Work out the finished part from the listing and answer in its coordinate system (mm). Face numbers are marked on the shaded views. A direction names the side the tool comes from. Give positions to 0.01 mm unless a question says otherwise; leave off trailing zeros. Loops run counter-clockwise (first coordinate to the right, second up) from the corner with the lowest first, then second, coordinate; pieces in that order, holes last. Notation, with made-up numbers: (63, 65) - (112, 65) arc R15 ccw to (112, 71) - close; hole circle Ø3 at (54.5, -2.75). An arc over 180 degrees is marked (long way). One line per item, written item: value.
from build123d import *

# Parameters (mm, degrees)
PROFILE_EXTRUDE_DEPTH                = 80
SPROCKET_SKETCH_R                    = 0.35
SPROCKET_EXTRUDE_DEPTH               = 1
SPROCKET_PATTERN_COUNT               = 7
SPROCKET_PATTERN_PITCH               = 12
MAGNET_START                         = -6.5
MAGNET_CUT_DEPTH                     = 5
MAGNET_CHAMFER_SIZE                  = 0.75
MAGNET_CHAMFER_OF_MAGNET_MIRROR_SIZE = 0.75


with BuildPart() as part:
    # Profile Sketch → Profile Extrude (new body)
    with BuildSketch(Plane(origin=(0.045617437, 0, -0.024209872), x_dir=(-1, 0, 0), z_dir=(0, 1, 0))):
        Polygon((3.545617437, -11.975790128), (3.545617437, 0.024209872), (-0.104382563, 0.024209872), (-0.104382563, 1.024209872), (-0.954382563, 1.024209872), (-0.954382563, -18.475790128), (13.045617437, -18.475790128), (13.045617437, 1.024209872), (12.195617437, 1.024209872), (12.195617437, 0.024209872), (10.795617437, 0.024209872), (10.795617437, -11.975790128), align=None)
    extrude(amount=PROFILE_EXTRUDE_DEPTH)

    # Sprocket Sketch → Sprocket Extrude (add)
    with BuildSketch(Plane.XY):
        with Locations(Location((-1.75, 2, 0), (0, 0, 180))):
            Circle(SPROCKET_SKETCH_R)
    sprocket_extrude = extrude(amount=SPROCKET_EXTRUDE_DEPTH)

    # Sprocket Pattern: Sprocket Extrude ×7
    with Locations(*[(0, i * SPROCKET_PATTERN_PITCH, 0) for i in range(1, SPROCKET_PATTERN_COUNT)]):
        add(sprocket_extrude)

    # Magnet Hole Sketch → Magnet Cut (cut)
    with BuildSketch(Plane.XY.offset(-12).offset(MAGNET_START)):
        with BuildLine():
            ThreePointArc((-5.276039281, 12.971757773), (-6.369559557, 12.644203044), (-7.125, 13.5))
            ThreePointArc((-7.125, 13.5), (-8.753920776, 14.461963369), (-9.379949311, 12.676789795))
            ThreePointArc((-9.379949311, 12.676789795), (-9.4063426, 11.535570233), (-10.453697807, 11.08155948))
            ThreePointArc((-10.453697807, 11.08155948), (-11.87194354, 9.829626791), (-10.367596036, 8.682589301))
            ThreePointArc((-10.367596036, 8.682589301), (-9.29038771, 8.304831552), (-9.182248383, 7.16844052))
            ThreePointArc((-9.182248383, 7.16844052), (-8.429851675, 5.432740197), (-6.874085251, 6.509005616))
            ThreePointArc((-6.874085251, 6.509005616), (-6.181940604, 7.41675805), (-5.067751617, 7.16844052))
            ThreePointArc((-5.067751617, 7.16844052), (-3.184499145, 7.347651415), (-3.727330121, 9.159857515))
            ThreePointArc((-3.727330121, 9.159857515), (-4.37676953, 10.098637121), (-3.796302193, 11.08155948))
            ThreePointArc((-3.796302193, 11.08155948), (-3.384784865, 12.928018228), (-5.276039281, 12.971757773))
        make_face()
    magnet_cut = extrude(amount=MAGNET_CUT_DEPTH, mode=Mode.SUBTRACT)

    # Magnet Chamfer
    magnet_chamfer_edges = [part.edges().sort_by_distance(p)[0] for p in [
        (-3.384784865, 12.928018228, -18.5),
        (-8.753920776, 14.461963369, -18.5),
        (-11.87194354, 9.829626791, -18.5),
        (-8.429851675, 5.432740197, -18.5),
        (-3.184499145, 7.347651415, -18.5),
        (-4.37676953, 10.098637121, -18.5),
        (-6.181940604, 7.41675805, -18.5),
        (-9.29038771, 8.304831552, -18.5),
        (-9.4063426, 11.535570233, -18.5),
        (-6.369559557, 12.644203044, -18.5),
    ]]
    chamfer(magnet_chamfer_edges, length=MAGNET_CHAMFER_SIZE)

    # Magnet Mirror: Magnet Cut across plane
    add(magnet_cut.mirror(Plane(origin=(0, 40, 0), x_dir=(0, 0, 1), z_dir=(0, -1, 0))), mode=Mode.SUBTRACT)

    # Magnet Chamfer of Magnet Mirror
    magnet_chamfer_of_magnet_mirror_edges = [part.edges().sort_by_distance(p)[0] for p in [
        (-3.384784865, 67.071981772, -18.5),
        (-8.753920776, 65.538036631, -18.5),
        (-11.87194354, 70.170373209, -18.5),
        (-8.429851675, 74.567259803, -18.5),
        (-3.184499145, 72.652348585, -18.5),
        (-4.37676953, 69.901362879, -18.5),
        (-6.181940604, 72.58324195, -18.5),
        (-9.29038771, 71.695168448, -18.5),
        (-9.4063426, 68.464429767, -18.5),
        (-6.369559557, 67.355796956, -18.5),
    ]]
    chamfer(magnet_chamfer_of_magnet_mirror_edges, length=MAGNET_CHAMFER_OF_MAGNET_MIRROR_SIZE)


solid = part.part
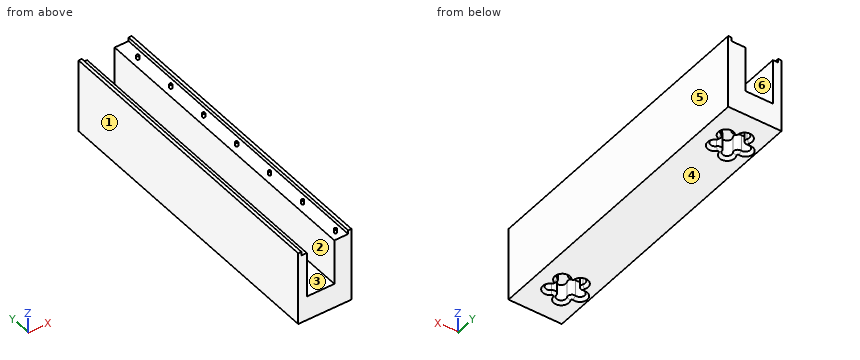
1. Flat-ended cylindrical pins translate along their axes: pin 1 Ø2 at (x, z) = (-9.5, -4.5) entering from +Y; pin 2 Ø1.5 at (x, y) = (-10.65, 70.13) entering from +Z; pin 3 Ø6 at (x, y) = (-7.5, 30.5) entering from +Z; pin 4 Ø2.5 at (x, y) = (-9.5, 10) entering from -Z. Find the tip coordinate at first contact, or state that the pin passes through.
Output:
pin 1: passes through
pin 2: stops at z = 0
pin 3: stops at z = -12
pin 4: stops at z = -17.79
2. Section B-B (y = 47.5) is taken. Write down the section's boundary in (x, z), and give its area (3 significant figures).
Output:
outline: (-13, -18.5) - (1, -18.5) - (1, 1) - (0.15, 1) - (0.15, 0) - (-3.5, 0) - (-3.5, -12) - (-10.75, -12) - (-10.75, 0) - (-12.15, 0) - (-12.15, 1) - (-13, 1) - close
area: 174 mm²
3. Section A-A (z = -7.25) is taken. Write down the section's boundary in (x, y), and give its area (3 significant figures).
Output:
outline: (-13, 0) - (-10.75, 0) - (-10.75, 80) - (-13, 80) - close; (-3.5, 0) - (1, 0) - (1, 80) - (-3.5, 80) - close
area: 540 mm²
4. The mould has two halves that part along X. Classify the marked faces 3, 4, 5 and 6: released by +X, released by -X, zero draft, split by the parting line, or undercut.
Output:
face 3: undercut
face 4: zero draft
face 5: released by +X
face 6: undercut
5. For the marked faces 1 and 2, determine the directions among +Z, -Z, +X, -X, +Y, -Y from which every point of the face is accessible in a straight line to the end or side of a thin tool.
Output:
face 1: +Z, -Z, -X, +Y, -Y
face 2: +Z, +Y, -Y
6. Section C-C (z = -14.5) is taken. Write down the section's boundary in (x, y) (3 decimals).
Output:
outline: (-13, 0) - (1, 0) - (1, 80) - (-13, 80) - close; hole (-10.454, 11.082) arc R1.224 ccw (long way) to (-10.368, 8.683) arc R1.059 cw to (-9.182, 7.168) arc R1.224 ccw (long way) to (-6.874, 6.509) arc R1.059 cw to (-5.068, 7.168) arc R1.224 ccw (long way) to (-3.727, 9.16) arc R1.059 cw to (-3.796, 11.082) arc R1.224 ccw (long way) to (-5.276, 12.972) arc R1.059 cw to (-7.125, 13.5) arc R1.224 ccw (long way) to (-9.38, 12.677) arc R1.059 cw to start; hole (-10.454, 68.918) arc R1.059 cw to (-9.38, 67.323) arc R1.224 ccw (long way) to (-7.125, 66.5) arc R1.059 cw to (-5.276, 67.028) arc R1.224 ccw (long way) to (-3.796, 68.918) arc R1.059 cw to (-3.727, 70.84) arc R1.224 ccw (long way) to (-5.068, 72.832) arc R1.059 cw to (-6.874, 73.491) arc R1.224 ccw (long way) to (-9.182, 72.832) arc R1.059 cw to (-10.368, 71.317) arc R1.224 ccw (long way) to start
7. Find the intervals of material crossed by line 1 along X through (y, z) = (50, 0.25); line 2 along X through (y, z) = (41, -0.5); line 3 along Z through (x, y) = (-3, 56.5), in increasing order.
Output:
line 1: x = -13 to -12.15, -2.1 to -1.4, 0.15 to 1
line 2: x = -13 to -10.75, -3.5 to 1
line 3: z = -18.5 to 0
